Work out the finished part from the listing and answer in its coordinate system (mm). A direction names the side the tool comes from. Round coordinates to 2 decimals unless told otherwise and drop trailing zeros. Write each loop counter-clockwise with the first axis right and the second up, starting at its lowest first coordinate (ties: lowest second). Pieces come first, ordered by that corner, then holes. Notation, with made-up numbers: (56, 86.5) -> (69, 86.5) arc R24 ccw to (69, 116.5) -> close; hole circle Ø3 at (28, 67.5). An arc over 180 degrees is marked (long way). One line per question, with ' | ' between items. Start each with the question number.
```python
from build123d import *

# Parameters (mm, degrees)
F1_DEPTH = 50
F3_DEPTH = 15
F5_DEPTH = 15
F6_R     = 4
F7_DEPTH = 90
F6_R_2   = 2.5
F8_DEPTH = 15


with BuildPart() as f1:
    # F0 (on Top) → F1 (new body)
    with BuildSketch(Plane.XY):
        Polygon((144, 38.584684), (105.415316, 105.415316), (60, 131.635861), (60, 174), (-60, 174), (-60, 131.635861), (-105.415316, 105.415316), (-144, 38.584684), (-144, -38.584684), (-105.415316, -105.415316), (-38.584684, -144), (38.584684, -144), (105.415316, -105.415316), (144, -38.584684), align=None)
    extrude(amount=F1_DEPTH)

    # F2 (on face) → F3 (cut)
    with BuildSketch(Plane.XY.offset(50)):
        with BuildLine():
            Line((-40, 159), (-60, 159))
            Line((-60, 159), (-60, 144))
            Line((-60, 144), (-40, 144))
            ThreePointArc((-40, 144), (-32.5, 151.5), (-40, 159))
        make_face()
        with BuildLine():
            Line((60, 144), (60, 159))
            Line((60, 159), (40, 159))
            ThreePointArc((40, 159), (32.5, 151.5), (40, 144))
            Line((40, 144), (60, 144))
        make_face()
    extrude(amount=-F3_DEPTH, mode=Mode.SUBTRACT)

    # F4 (on face) → F5 (cut)
    with BuildSketch(Plane.XY):
        with BuildLine():
            Line((60, 144), (60, 159))
            Line((60, 159), (40, 159))
            ThreePointArc((40, 159), (32.5, 151.5), (40, 144))
            Line((40, 144), (60, 144))
        make_face()
        with BuildLine():
            Line((-40, 159), (-60, 159))
            Line((-60, 159), (-60, 144))
            Line((-60, 144), (-40, 144))
            ThreePointArc((-40, 144), (-32.5, 151.5), (-40, 159))
        make_face()
    extrude(amount=F5_DEPTH, mode=Mode.SUBTRACT)

    # F6 (on face) → F7 (cut)
    with BuildSketch(Plane(origin=(0, 174, 0), x_dir=(-1, 0, 0), z_dir=(0, 1, 0))):
        with Locations((-50, 25)):
            Circle(F6_R)
        with Locations((50, 25)):
            Circle(F6_R)
    extrude(amount=-F7_DEPTH, mode=Mode.SUBTRACT)

    # F6 (on face) → F8 (cut, through all)
    with BuildSketch(Plane(origin=(0, 174, 0), x_dir=(-1, 0, 0), z_dir=(0, 1, 0))):
        with Locations((-50, 42.5)):
            Circle(F6_R_2)
        with Locations((-50, 7.5)):
            Circle(F6_R_2)
        with Locations((50, 7.5)):
            Circle(F6_R_2)
        with Locations((50, 42.5)):
            Circle(F6_R_2)
    extrude(amount=-F8_DEPTH, mode=Mode.SUBTRACT)


solid = f1.part
```
(1) A cutting plane is placed at C-C, the plane x = -65. Determine the outline of the cut face in (y, z).
(2) A cutting plane is placed at B-B, the plane z = 25. Determine the outline of the cut face in (x, y).
(3) A cutting plane is placed at A-A, the plane y = 151.5. Determine the outline of the cut face in (x, z), then the cut area to 3 significant figures.
(4) Consider L1, parallel to Z at x = -50, y = 167.5; L2, parallel to Z at x = 50, y = 130.5; L3, parallel to X at y = 89, z = 28.5. Determine where each line is inside the solid, lowest interval first.
(5) Given pin 1 Ø7.5 at (x, z) = (-45, 39) entering from -Y; pin 2 Ø10 at (x, y) = (-86, 119) entering from -Z; pin 3 Ø7.5 at (x, y) = (49, 148) entering from +Z; pin 4 Ø10 at (y, z) = (116, 8) entering from -X, each flat-ended and moving along its own axis, determine where each tip first touches the part or whether it passes through.
(6) For faces 5 (the cylindrical face through (52.95, 129.63, 27.7)), 6 (the flat face through (46, 152, 15)), 7 (the flat face through (-47.6, 159, 9.1)), 8 (the flat face through (47.9, 159, 44.3)), 9 (the flat face through (60, 153, 25)), determine the directions among +Z, -Z, +X, -X, +Y, -Y from which every point of the face is accessible in a straight line to the end or side of a thin tool.
(7) The mould has two halves that part along Z. Classify faces 1 (the flat face through (-2, 17, 50)), 2 (the flat face through (-50, 84, 25)), 3 (the flat face through (-2, 17, 0)), 4 (the cylindrical face through (-32.5, 151.34, 7.4)): +Z half, -Z half, draft (parallel to the pull), parting line (faces both ways), or undercut.
Returned:
1) outline: (-128.75, 0) -> (128.75, 0) -> (128.75, 50) -> (-128.75, 50) -> close
2) outline: (-144, -38.58) -> (-105.42, -105.42) -> (-38.58, -144) -> (38.58, -144) -> (105.42, -105.42) -> (144, -38.58) -> (144, 38.58) -> (105.42, 105.42) -> (60, 131.64) -> (60, 174) -> (54, 174) -> (54, 84) -> (46, 84) -> (46, 174) -> (-46, 174) -> (-46, 84) -> (-54, 84) -> (-54, 174) -> (-60, 174) -> (-60, 131.64) -> (-105.42, 105.42) -> (-144, 38.58) -> close
3) outline: (-60, 15) -> (-32.5, 15) -> (-32.5, 0) -> (32.5, 0) -> (32.5, 15) -> (60, 15) -> (60, 35) -> (32.5, 35) -> (32.5, 50) -> (-32.5, 50) -> (-32.5, 35) -> (-60, 35) -> close; hole circle Ø8 at (-50, 25); hole circle Ø8 at (50, 25) | area: 4,250 mm2
4) L1: 0 to 5, 10 to 21, 29 to 40, 45 to 50 | L2: 0 to 21, 29 to 50 | L3: -114.89 to -51.94, -48.06 to 48.06, 51.94 to 114.89
5) pin 1: y = -142.46 | pin 2: z = 0 | pin 3: z = 35 | pin 4: x = -95.74
6) face 5: +Y | face 6: -Z, +X | face 7: -Z, -X | face 8: +Z, +X | face 9: +Z, -Z, +X, +Y
7) face 1: +Z half | face 2: undercut | face 3: -Z half | face 4: draft
